```python
from build123d import *

# Parameters (mm, degrees)
F0_R     = 1.75
F1_DEPTH = 25
F3_DEPTH = 12.5


with BuildPart() as f1:
    # F0 (on Top) → F1 (new body)
    with BuildSketch(Plane.XY):
        with BuildLine():
            Line((3.980159, 0.397914), (3.980159, 154.602086))
            ThreePointArc((3.980159, 154.602086), (0, 159), (-3.980159, 154.602086))
            Line((-3.980159, 154.602086), (-3.980159, 0.397914))
            ThreePointArc((-3.980159, 0.397914), (0, -4), (3.980159, 0.397914))
        make_face()
        Circle(F0_R, mode=Mode.SUBTRACT)
        with Locations((0, 155)):
            Circle(F0_R, mode=Mode.SUBTRACT)
    extrude(amount=F1_DEPTH)

    # F2 (on Right) → F3 (intersect, symmetric)
    with BuildSketch(Plane.YZ):
        with BuildLine():
            Line((-4, 0), (0, 0))
            Line((0, 0), (4, 0))
            ThreePointArc((4, 0), (77.5, 1.351019), (151, 0))
            Line((151, 0), (159, 0))
            Line((159, 0), (159, 3))
            Line((159, 3), (151, 3))
            Line((151, 3), (151, 12))
            Line((151, 12), (159, 12))
            Line((159, 12), (159, 15))
            Line((159, 15), (151, 15))
            ThreePointArc((151, 15), (77.5, 13.648981), (4, 15))
            Line((4, 15), (-4, 15))
            Line((-4, 15), (-4, 12))
            Line((-4, 12), (4, 12))
            Line((4, 12), (4, 3))
            Line((4, 3), (-4, 3))
            Line((-4, 3), (-4, 0))
        make_face()
    extrude(amount=F3_DEPTH, both=True, mode=Mode.INTERSECT)


solid = f1.part
```
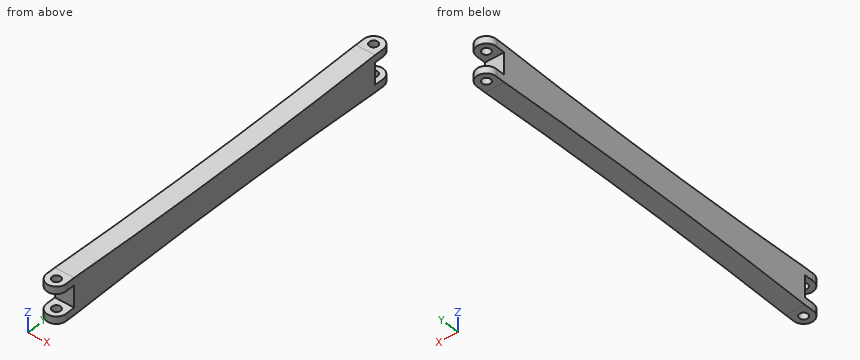
Input: part model. Units: mm. Frame: model coordinates. Give positions to 0.01 mm unless a question says otherwise; leave off trailing zeros. Order: outer loops, then holes, each group sorted by start corner. A loop starts at its lowest first (then second) coordinate and runs counter-clockwise, first axis right, second up. Notation, with made-up numbers: M 46,15.25 L 64,15.25 A13 ccw 64,38.25 Z; hole C 41.5,31 d8. An arc over 180 degrees is marked long. Return JSON: item names as keys, results as strings.
1) Section query C-C on y = 76. Output: boundary loops of the cut face in (x, z), and give its area (3 significant figures).
Taken from the geometry:
{"outline": "M -3.98,1.35 L 3.98,1.35 L 3.98,13.65 L -3.98,13.65 Z", "area": "97.9 mm2"}
2) Section query B-B on z = 5.5. Output: boundary loops of the cut face in (x, y).
Taken from the geometry:
{"outline": "M -3.98,4 L 3.98,4 L 3.98,151 L -3.98,151 Z"}
3) Contact query for flat-ended pins moving along their axis: pin 1 (8 mm diameter, centred on y = 20.5, z = 3.5, fed in from -X); pin 2 (2 mm diameter, centred on x = 0, y = 155, fed in from -Z); pin 3 (4 mm diameter, centred on x = 2, z = 9, fed in from +Y); pin 4 (6 mm diameter, centred on y = 100.5, z = 7, fed in from +X). Output: stop coordinate, or through.
Taken from the geometry:
{"pin 1": "stops at x = -3.98", "pin 2": "passes through", "pin 3": "stops at y = 151", "pin 4": "stops at x = 3.98"}
4) Section query A-A on x = 0. Count the separate pieces of the cut face and the enclosed holes in it, and give its area (3 significant figures).
Taken from the geometry:
{"separate pieces": "5", "enclosed holes": "0", "area": "1,990 mm2"}
5) Line query: L1, parallel to Y at x = 0.25, z = 12.75; L2, parallel to Z at x = 3.5, y = 3.5; L3, parallel to X at y = 0, z = 2.25. Output: solid intervals per line, ascending. Write a range as [from, to].
Taken from the geometry:
{"L1": "y = [-3.99, -1.73], [1.73, 153.27], [156.73, 158.99]", "L2": "z = [0, 3], [12, 15]", "L3": "x = [-4, -1.75], [1.75, 4]"}
